```python
from build123d import *

# Parameters (mm, degrees)
SKETCH1_R            = 7.5
BOSS_EXTRUDE1_DEPTH  = 67.685
CUT_EXTRUDE2_DEPTH   = 69.511015355
CUT_EXTRUDE3_DEPTH   = 69.511015476
SKETCH8_R            = 3
CUT_EXTRUDE4_DEPTH   = 69.903985677
FILLET1_R            = 1
FILLET1_OF_MIRROR2_R = 1


with BuildPart() as part:
    # Sketch1 → Boss-Extrude1 (new, symmetric)
    with BuildSketch(Plane.XY):
        Circle(SKETCH1_R)
    extrude(amount=BOSS_EXTRUDE1_DEPTH, both=True)

    # Sketch6 → Cut-Extrude2 (cut, symmetric)
    with BuildSketch(Plane(origin=(0, 0, 0), x_dir=(0, 0, -1), z_dir=(1, 0, 0))):
        with BuildLine():
            Line((67.685, 0), (67.685, 7.5))
            Line((67.685, 7.5), (61.685, 7.5))
            ThreePointArc((61.685, 7.5), (66.000428973, 4.802343178), (67.685, 0))
        make_face()
        with BuildLine():
            Line((67.685, -7.5), (67.685, 0))
            ThreePointArc((67.685, 0), (66.000428973, -4.802343178), (61.685, -7.5))
            Line((61.685, -7.5), (67.685, -7.5))
        make_face()
    cut_extrude2 = extrude(amount=CUT_EXTRUDE2_DEPTH, both=True, mode=Mode.SUBTRACT)

    # Sketch7 → Cut-Extrude3 (cut, symmetric)
    with BuildSketch(Plane(origin=(0, 0, 0), x_dir=(1, 0, 0), z_dir=(0, 1, 0))):
        Polygon((-3, 67.685), (-3, 52.685), (-7.5, 51.891528587), (-7.5, 67.685), align=None)
        Polygon((7.5, 67.685), (3, 67.685), (3, 52.685), (7.5, 51.891528587), align=None)
    cut_extrude3 = extrude(amount=CUT_EXTRUDE3_DEPTH, both=True, mode=Mode.SUBTRACT)

    # Sketch8 → Cut-Extrude4 (cut, symmetric)
    with BuildSketch(Plane(origin=(-3, 0, 0), x_dir=(0, 0, -1), z_dir=(1, 0, 0))):
        with Locations((59.9975, 0)):
            Circle(SKETCH8_R)
    cut_extrude4 = extrude(amount=CUT_EXTRUDE4_DEPTH, both=True, mode=Mode.SUBTRACT)

    # Fillet1
    fillet1_edges = [part.edges().sort_by_distance(p)[0] for p in [
        (-3, 0, -52.685),
        (3, 0, -52.685),
    ]]
    fillet(fillet1_edges, radius=FILLET1_R)

    # Mirror2: Cut-Extrude2, Cut-Extrude3, Cut-Extrude4 across plane
    add(cut_extrude2.mirror(Plane.XY), mode=Mode.SUBTRACT)
    add(cut_extrude3.mirror(Plane.XY), mode=Mode.SUBTRACT)
    add(cut_extrude4.mirror(Plane.XY), mode=Mode.SUBTRACT)

    # Fillet1 of Mirror2
    fillet1_of_mirror2_edges = [part.edges().sort_by_distance(p)[0] for p in [
        (-3, 0, 52.685),
        (3, 0, 52.685),
    ]]
    fillet(fillet1_of_mirror2_edges, radius=FILLET1_OF_MIRROR2_R)


solid = part.part
```
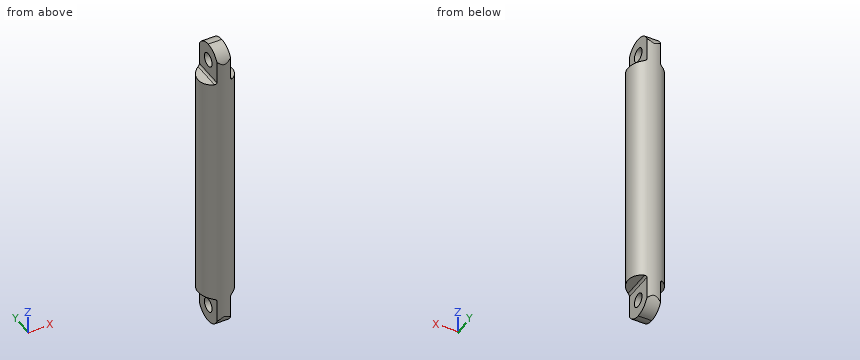
Model file for the job. Use its own axes, mm. Coordinates: 2 decimals unless noted, no trailing zeros. Order: outer loops, then holes, each group sorted by start corner. A loop starts at its lowest first (then second) coordinate and runs counter-clockwise, first axis right, second up. Notation, with made-up numbers: (9, 70) -> (68, 70) arc R22 cw to (68, 102) -> close; hole circle Ø2 at (-3.5, 34). An arc over 180 degrees is marked (long way). Answer as a JSON object with one key per item and string values. Group by question number.
1) Cut at A-A, the plane x = 0. Write the cut outline in (y, z) (1 decimal).
2) Cut at D-D, the plane y = -5. Write the cut outline in (x, z), then the cut area to 3 significant figures.
3) Cut at C-C, the plane z = 42. Write the cut outline in (x, y), then the cut area to 3 significant figures.
4) Drill centre lines: L1, parallel to Z at x = -1.5, y = -1; L2, parallel to Z at x = -0.5, y = 2.5; L3, parallel to Y at x = 4.25, z = 8. Where is each one in solid material? Low to high.
5) Flat gauge pins, fed straight in: pin 1 (1 mm diameter, centred on y = 2.5, z = -34, fed in from +X); pin 2 (7 mm diameter, centred on y = -1, z = 57.5, fed in from +X); pin 3 (1 mm diameter, centred on x = 0.5, y = 3, fed in from +Z). Where does each tip first touch, or does it go through?
6) Cut at B-B, the plane y = 1.75. Write the cut outline in (x, z).
Check values:
{
 "1": {"outline": "(-7.5, -61.7) arc R7.7 ccw to (7.5, -61.7) -> (7.5, 61.7) arc R7.7 ccw to (-7.5, 61.7) -> close; hole circle Ø6 at (0, -60); hole circle Ø6 at (0, 60)"},
 "2": {"outline": "(-5.59, -52.23) -> (-3.83, -52.54) arc R1 cw to (-3, -53.52) -> (-3, -65.84) -> (3, -65.84) -> (3, -53.52) arc R1 cw to (3.83, -52.54) -> (5.59, -52.23) -> (5.59, 52.23) -> (3.83, 52.54) arc R1 cw to (3, 53.52) -> (3, 65.84) -> (-3, 65.84) -> (-3, 53.52) arc R1 cw to (-3.83, 52.54) -> (-5.59, 52.23) -> close", "area": "1,330 mm²"},
 "3": {"outline": "circle Ø15 at (0, 0)", "area": "177 mm²"},
 "4": {"L1": "z = -67.62 to -62.83, -57.17 to 57.17, 62.83 to 67.62", "L2": "z = -67.27 to -61.66, -58.34 to 58.34, 61.66 to 67.27", "L3": "y = -6.18 to 6.18"},
 "5": {"pin 1": "stops at x = 7.23", "pin 2": "stops at x = 3", "pin 3": "stops at z = 67.27"},
 "6": {"outline": "(-7.29, -51.93) -> (-3.83, -52.54) arc R1 cw to (-3, -53.52) -> (-3, -57.56) -> (3, -57.56) -> (3, -53.52) arc R1 cw to (3.83, -52.54) -> (7.29, -51.93) -> (7.29, 51.93) -> (3.83, 52.54) arc R1 cw to (3, 53.52) -> (3, 57.56) -> (-3, 57.56) -> (-3, 53.52) arc R1 cw to (-3.83, 52.54) -> (-7.29, 51.93) -> close; (-3, -67.48) -> (3, -67.48) -> (3, -62.43) -> (-3, -62.43) -> close; (-3, 62.43) -> (3, 62.43) -> (3, 67.48) -> (-3, 67.48) -> close"}
}
